```python
from build123d import *

# Parameters (mm, degrees)
F0_W          = 39.99992
F0_H          = 39.99992
F1_DEPTH      = 12.7
F3_D          = 3.6576
F3_DEPTH      = 7.62
F3_TIP        = 1.0988539001
F4_W          = 39.99992
F4_H          = 12.7
F5_DEPTH      = 39.99992
F6_W          = 39.99992
F6_H          = 39.99992
F7_DEPTH      = 22.14626
F7_DEPTH_BACK = 3.048
F8_W          = 12.49426
F8_H          = 13.64996
F9_DEPTH      = 39.99992
F10_R         = 5.08
F12_D         = 3.6576
F12_DEPTH     = 7.62
F12_TIP       = 1.0988539001
F14_DEPTH     = 25.4


with BuildPart() as f1:
    # F0 (on Top) → F1 (new body)
    with BuildSketch(Plane.XY):
        Rectangle(F0_W, F0_H)
    extrude(amount=F1_DEPTH)

    # F3
    with Locations(Plane(origin=(0, 0, 0), x_dir=(1, 0, 0), z_dir=(0, 0, -1))):
        with Locations((-15.875, -15.875), (15.875, -15.875), (15.875, 15.875), (-15.875, 15.875)):
            Hole(F3_D / 2, depth=F3_DEPTH)
            with Locations((0, 0, -(F3_DEPTH + F3_TIP / 2))):  # 118° drill point
                Cone(0, F3_D / 2, F3_TIP, mode=Mode.SUBTRACT)

    # F4 (on face) → F5 (join)
    with BuildSketch(Plane.XY.offset(12.7)):
        Rectangle(F4_W, F4_H)
    extrude(amount=F5_DEPTH)

    # F6 (on face) → F7 (join, two sides)
    with BuildSketch(Plane(origin=(-19.99996, 0, 0), x_dir=(0, -1, 0), z_dir=(-1, 0, 0))) as f7_sk:
        with Locations((0, 32.69996)):
            Rectangle(F6_W, F6_H)
    extrude(amount=F7_DEPTH)
    extrude(f7_sk.sketch, amount=-F7_DEPTH_BACK)

    # F8 (on face) → F9 (cut)
    with BuildSketch(Plane.XY.offset(52.69992)):
        with Locations((-23.19909, 13.17498)):
            Rectangle(F8_W, F8_H)
        with Locations((-23.19909, -13.17498)):
            Rectangle(F8_W, F8_H)
    extrude(amount=-F9_DEPTH, mode=Mode.SUBTRACT)

    # F10
    f10_edges = [f1.edges().sort_by_distance(p)[0] for p in [
        (-29.44622, -6.35, 32.69996),
        (-29.44622, 6.35, 32.69996),
    ]]
    fillet(f10_edges, radius=F10_R)

    # F12
    with Locations(Plane(origin=(-42.14622, 0, 0), x_dir=(0, -1, 0), z_dir=(-1, 0, 0))):
        with Locations((-15.875, 48.57496), (15.875, 48.57496), (15.875, 16.82496), (-15.875, 16.82496)):
            Hole(F12_D / 2, depth=F12_DEPTH)
            with Locations((0, 0, -(F12_DEPTH + F12_TIP / 2))):  # 118° drill point
                Cone(0, F12_D / 2, F12_TIP, mode=Mode.SUBTRACT)

    # F13 (on face) → F14 (cut, symmetric)
    with BuildSketch(Plane.XZ.offset(6.35)):
        Polygon((-29.44622, 52.69992), (-24.36622, 48.5904095464), (-24.36622, 52.69992), align=None)
        Polygon((-24.36622, 48.5904095464), (19.99996, 12.7), (19.99996, 52.69992), (-24.36622, 52.69992), align=None)
    extrude(amount=F14_DEPTH, both=True, mode=Mode.SUBTRACT)


solid = f1.part
```
Source: CAD feature listing. Evaluate the final solid. Frame: model axes, mm. A direction names the side the tool comes from. Coordinates: 2 decimals unless noted, no trailing zeros. Write each loop counter-clockwise with the first axis right and the second up, starting at its lowest first coordinate (ties: lowest second). Pieces come first, ordered by that corner, then holes. Notation, with made-up numbers: (-18.5, 3) -> (-14.5, 3) arc R23 ccw to (-14.5, 39) -> close; hole circle Ø8 at (32, 57). An arc over 180 degrees is marked (long way). Return JSON: item names as keys, results as strings. Group by question number.
1) Contact query for flat-ended pins moving along their axis: P1, Ø3, axis at y = -15.88, z = 16.82, coming from the -X side; P2, Ø4, axis at x = -5, y = 13.5, coming from the +Z side; P3, Ø2, axis at y = 15.88, z = 48.57, coming from the -X side. Output: stop coordinate, or through.
2) Section query B-B, the plane z = 4. Return loops of the section in (x, y) (3 decimals), plus the area to 3 significant figures.
3) Section query A-A, the plane y = -13. Return loops of the section in (x, z).
4) Section query C-C, the plane x = -36. Return loops of the section in (y, z) (3 decimals), plus the area to 3 significant figures.
5) Ray query, line 1 along Z through (x, y) = (10, 10.5); line 2 along X through (y, z) = (11, 29); line 3 along Y through (x, z) = (-5.5, 32.5). Return the intervals inside material, ascending.
6) Section query D-D, the plane y = -1.5. Return loops of the section in (x, z).
7) Set-up query: faces 1 (the face through (-29.446, -16, 33)), 2 (the face through (-20, 0, 6)), 3 (the face through (-38.28, 15.64, 50.39)). Return all of +Z, -Z, +X, -X, +Y, -Y with unobstructed straight access to the full face (end or side cutting, diameter ignored); none if empty.
8) Mould query, pull axis Y, two halves, no side actions, for faces 4 (the face through (-36, -20, 32)), 5 (the face through (-33.6, 15.7, 48.8)), 6 (the face through (-36, 0, 52.7)), 7 (the face through (15.031, 17.497, 3.863)). Classes: +Y half, -Y half, draft (parallel to the pull), parting line (faces both ways), or undercut.
From the geometry:
{
 "1": {"P1": "x = -34.33", "P2": "z = 12.7", "P3": "x = -34.03"},
 "2": {"outline": "(-20, -20) -> (20, -20) -> (20, 20) -> (-20, 20) -> close; hole circle Ø3.658 at (-15.875, -15.875); hole circle Ø3.658 at (-15.875, 15.875); hole circle Ø3.658 at (15.875, -15.875); hole circle Ø3.658 at (15.875, 15.875)", "area": "1,560 mm²"},
 "3": {"outline": "(-42.15, 12.7) -> (-29.45, 12.7) -> (-29.45, 52.7) -> (-42.15, 52.7) -> close; (-20, 0) -> (20, 0) -> (20, 12.7) -> (-20, 12.7) -> close"},
 "4": {"outline": "(-20, 12.7) -> (20, 12.7) -> (20, 52.7) -> (-20, 52.7) -> close; hole circle Ø3.658 at (-15.875, 16.825); hole circle Ø3.658 at (-15.875, 48.575); hole circle Ø3.658 at (15.875, 16.825); hole circle Ø3.658 at (15.875, 48.575)", "area": "1,560 mm²"},
 "5": {"line 1": "0 to 12.7", "line 2": "-42.15 to -29.43", "line 3": "-6.35 to 6.35"},
 "6": {"outline": "(-42.15, 12.7) -> (-20, 12.7) -> (-20, 0) -> (20, 0) -> (20, 12.7) -> (-29.45, 52.7) -> (-42.15, 52.7) -> close"},
 "7": {"face 1": "+Z, -Z, +X, -Y", "face 2": "-Z, -X, +Y, -Y", "face 3": "-X"},
 "8": {"face 4": "-Y half", "face 5": "undercut", "face 6": "draft", "face 7": "undercut"}
}
